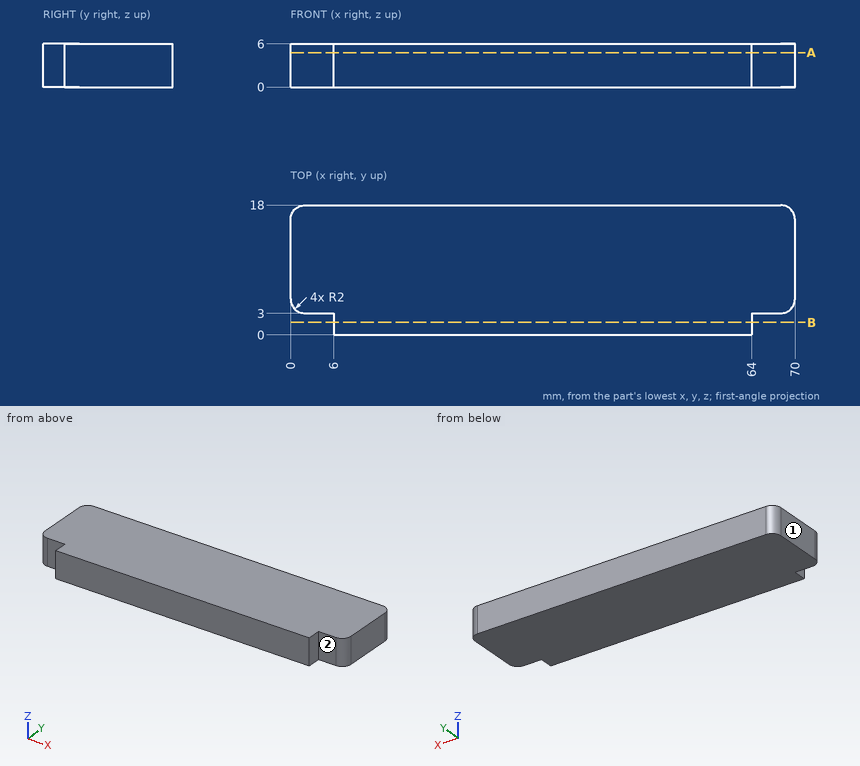
Geometry: see drawing. Coordinates: mm, zero at the bounding-box minimum. A direction names the side the tool comes from. Give positions to 0.01 mm unless a question says otherwise; leave off trailing zeros. Order: outer loops, then holes, each group sorted by start corner. A loop starts at its lowest first (then second) coordinate and runs counter-clockwise, first axis right, second up. Notation, with made-up numbers: (87.25, 18) - (137.25, 18) arc R28 ccw to (137.25, 50) - close; hole circle Ø9 at (88, 56). An arc over 180 degrees is marked (long way). Use a Markdown table: item, result.
(1) Access query for the marked faces 1 and 2. Directions: +Z, -Z, +X, -X, +Y, -Y. A direction counts if a zero-diameter tool reaches every point of the face in a straight line with its end or side. Return the directions, or none.
Computed values:
| item | result |
|---|---|
| face 1 | +Z, -Z, -X, +Y, -Y |
| face 2 | +Z, -Z, +X, -Y |
(2) Section query B-B (y = 1.75). Output: boundary loops of the cut face in (x, z).
Computed values:
| item | result |
|---|---|
| outline | (6, 0) - (64, 0) - (64, 6) - (6, 6) - close |
(3) Line query: line 1 (Y direction, x = 5, z = 1.6); line 2 (X direction, y = 17, z = 2.2); line 3 (X direction, y = 3.75, z = 1.75). Output: solid intervals per line, ascending. Write a range as from..to.
Computed values:
| item | result |
|---|---|
| line 1 | y = 3..18 |
| line 2 | x = 0.27..69.73 |
| line 3 | x = 0.44..69.56 |
(4) Section query A-A (z = 4.8). Output: boundary loops of the cut face in (x, y), then the cut area to 3 significant figures.
Computed values:
| item | result |
|---|---|
| outline | (0, 5) arc R2 ccw to (2, 3) - (6, 3) - (6, 0) - (64, 0) - (64, 3) - (68, 3) arc R2 ccw to (70, 5) - (70, 16) arc R2 ccw to (68, 18) - (2, 18) arc R2 ccw to (0, 16) - close |
| area | 1,220 mm2 |
(5) Pin query (flat end, axial travel): pin 1 (1.5 mm diameter, centred on x = 59, y = 6.5, fed in from -Z); pin 2 (2.5 mm diameter, centred on y = 2, z = 3, fed in from -X); pin 3 (3.5 mm diameter, centred on y = 2, z = 3, fed in from +X). Return the tip coordinate at first contact, or that it passes through.
Computed values:
| item | result |
|---|---|
| pin 1 | stops at z = 0 |
| pin 2 | stops at x = 1.03 |
| pin 3 | stops at x = 69.56 |
